Model file for the job. Use its own axes, mm. Face numbers are marked on the shaded views. A direction names the side the tool comes from. Round coordinates to 2 decimals unless told otherwise and drop trailing zeros. Order: outer loops, then holes, each group sorted by start corner. A loop starts at its lowest first (then second) coordinate and runs counter-clockwise, first axis right, second up. Notation, with made-up numbers: (52, 81) -> (108, 81) arc R37 cw to (108, 120) -> close; hole circle Ø2 at (84.5, -26). An arc over 180 degrees is marked (long way). Put each result on its own line as item: value. Start each with the question number.
Q1. Cut at A-A, the plane z = 0. List the corners of the cut face in (x, y).
Q2. Probe L1, parallel to Y at x = 25.6, z = 0; L2, parallel to X at y = -14, z = -0.5; L3, parallel to Y at x = 22, z = 0. List the from-to ranges inside material, lowest first.
Q3. Cut at D-D, the plane y = 8. State how many separate pieces and enclosed holes the cut face has, and give its area (3 significant figures).
Q4. Flat gauge pins, fed straight in: P1, Ø6, axis at x = 17.5, z = -11, coming from the +Y side; P2, Ø1.3, axis at x = 19.5, y = 4.5, coming from the -Z side; P3, Ø12, axis at x = 22, y = 8.5, coming from the +Z side; P4, Ø7.5, axis at y = 0, z = 0, coming from the -X side. Where does each tip first touch, or does it go through?
Q5. Cut at B-B, the plane y = 0. List the corners of the cut face in (x, z), and give its area (3 significant figures).
Q6. Cut at C-C, the plane x = 12.25. List the corners of the cut face in (y, z).
Q7. 3-axis set-ups, long thin cutter, end or side, ignore diameter. For the marked faces 1 and 2: which of +Z, -Z, +X, -X, +Y, -Y reach the whole face in a straight line?
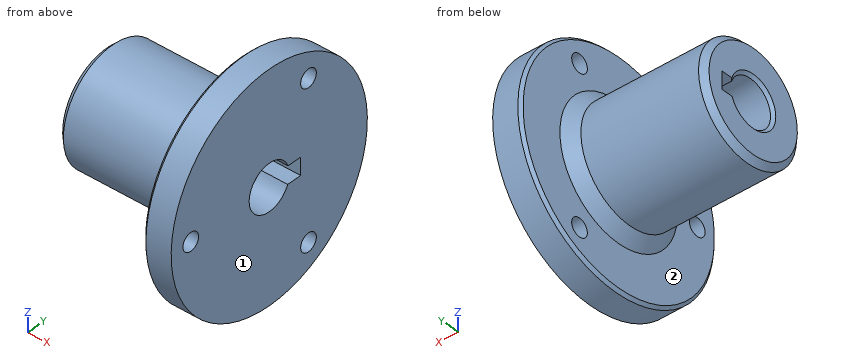
from build123d import *

# Parameters (mm, degrees)
SKETCH_1_R          = 10
EXTRUDE_1_DEPTH     = 24
SKETCH_2_R          = 20
SKETCH_2_R_2        = 1.6
EXTRUDE_2_DEPTH     = 5
CUT_EXTRUDE_1_REACH = 42.509
CHAMFER_1_SIZE      = 0.5
CHAMFER_2_SIZE      = 1
CHAMFER_3_SIZE      = 0.5
CHAMFER_4_SIZE      = 2


with BuildPart() as part:
    # 草图1 → 凸台-拉伸1 (new body)
    with BuildSketch(Plane(origin=(0, 0, 0), x_dir=(0, 0, -1), z_dir=(1, 0, 0))):
        Circle(SKETCH_1_R)
        with BuildLine():
            Line((-1.46, 6.008811728), (-1.46, 6.4))
            Line((-1.46, 6.4), (1.64, 6.4))
            Line((1.64, 6.4), (1.64, 6.008811728))
            Line((1.64, 6.008811728), (1.64, 3.75771207))
            ThreePointArc((1.64, 3.75771207), (-0.097219285, -4.098847205), (-1.46, 3.831240008))
            Line((-1.46, 3.831240008), (-1.46, 6.008811728))
        make_face(mode=Mode.SUBTRACT)
    extrude(amount=EXTRUDE_1_DEPTH)

    # 草图2 → 凸台-拉伸2 (add)
    with BuildSketch(Plane(origin=(24, 0, 0), x_dir=(0, 0, -1), z_dir=(1, 0, 0))):
        Circle(SKETCH_2_R)
        with Locations((-13.856406461, 8)):
            Circle(SKETCH_2_R_2, mode=Mode.SUBTRACT)
        with Locations((13.856406461, 8)):
            Circle(SKETCH_2_R_2, mode=Mode.SUBTRACT)
        with Locations((0, -16)):
            Circle(SKETCH_2_R_2, mode=Mode.SUBTRACT)
    extrude(amount=EXTRUDE_2_DEPTH)

    # 草图5 → 切除-拉伸1 (cut, up to next)
    with BuildSketch(Plane(origin=(29, 0, 0), x_dir=(0, 0, -1), z_dir=(1, 0, 0)), mode=Mode.PRIVATE) as cut_extrude_1_sk1:
        with BuildLine():
            Line((-1.46, 6.4), (-1.46, 3.831240008))
            ThreePointArc((-1.46, 3.831240008), (-0.097219285, -4.098847205), (1.64, 3.75771207))
            Line((1.64, 3.75771207), (1.64, 6.4))
            Line((1.64, 6.4), (-1.46, 6.4))
        make_face()
    cut_extrude_1_tool1 = extrude(cut_extrude_1_sk1.sketch, amount=-CUT_EXTRUDE_1_REACH, mode=Mode.PRIVATE) & part.part
    add(cut_extrude_1_tool1.solids().sort_by_distance((29, 0.642064, -0.012064))[0], mode=Mode.SUBTRACT)

    # 倒角1
    chamfer_1_edges = [part.edges().sort_by_distance(p)[0] for p in [
        (0, -4.098847205, 0.097219285),
    ]]
    chamfer(chamfer_1_edges, length=CHAMFER_1_SIZE)

    # 倒角2
    chamfer_2_edges = [part.edges().sort_by_distance(p)[0] for p in [
        (0, 0, 10),
    ]]
    chamfer(chamfer_2_edges, length=CHAMFER_2_SIZE)

    # 倒角3
    chamfer_3_edges = [part.edges().sort_by_distance(p)[0] for p in [
        (24, 0, 20),
    ]]
    chamfer(chamfer_3_edges, length=CHAMFER_3_SIZE)

    # 倒角4
    chamfer_4_edges = [part.edges().sort_by_distance(p)[0] for p in [
        (24, 0, 10),
    ]]
    chamfer(chamfer_4_edges, length=CHAMFER_4_SIZE)


solid = part.part
Ans:
1. outline: (0, -9) -> (1, -10) -> (22, -10) -> (24, -12) -> (24, -14.4) -> (29, -14.4) -> (29, -4.1) -> (0.5, -4.1) -> (0, -4.6) -> close; (0, 6.4) -> (29, 6.4) -> (29, 20) -> (24.5, 20) -> (24, 19.5) -> (24, 12) -> (22, 10) -> (1, 10) -> (0, 9) -> close; (24, -19.5) -> (24.5, -20) -> (29, -20) -> (29, -17.6) -> (24, -17.6) -> close
2. L1: y = -20 to -17.6, -14.4 to -4.1, 6.4 to 20
2. L2: x = 24 to 29
2. L3: y = -10 to -4.1, 6.4 to 10
3. separate pieces: 3
3. enclosed holes: 0
3. area: 443 mm^2
4. P1: stops at y = 6
4. P2: stops at z = -9.23
4. P3: stops at z = 19.77
4. P4: passes through
5. outline: (0, -9) -> (1, -10) -> (22, -10) -> (24, -12) -> (24, -19.5) -> (24.5, -20) -> (29, -20) -> (29, -4.1) -> (0.5, -4.1) -> (0, -4.6) -> close; (0, 4.6) -> (0.5, 4.1) -> (29, 4.1) -> (29, 20) -> (24.5, 20) -> (24, 19.5) -> (24, 12) -> (22, 10) -> (1, 10) -> (0, 9) -> close
5. area: 445 mm^2
6. outline: circle Ø20 at (0, 0); hole (3.76, -1.64) -> (6.4, -1.64) -> (6.4, 1.46) -> (3.83, 1.46) arc R4.1 ccw (long way) to start
7. face 1: +Z, -Z, +X, +Y, -Y
7. face 2: -X
